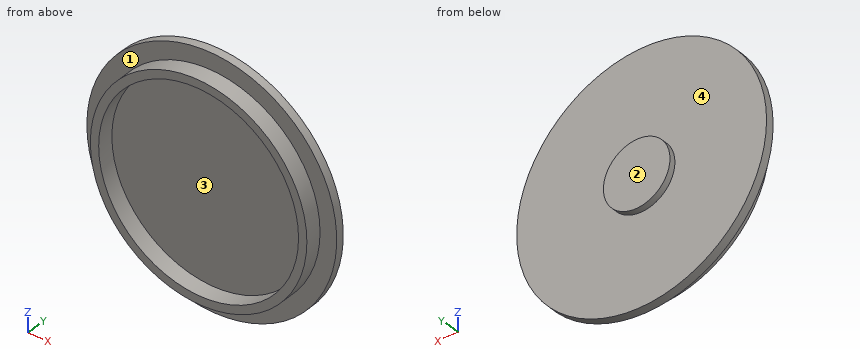
```python
from build123d import *


with BuildPart() as part:
    # Sketch1 → Lid Revolve (revolve)
    with BuildSketch(Plane.XY, mode=Mode.PRIVATE) as lid_revolve_sk:
        Polygon((0, 0), (48, 0), (48, -8), (52, -8), (52, 0), (60, 0), (60, 4), (16, 4), (16, 7), (0, 7), align=None)
    revolve(lid_revolve_sk.sketch.rotate(Axis((0, 7, 0), (0, -1, 0)), 180), axis=Axis((0, 7, 0), (0, -1, 0)))


solid = part.part
```
Input: part model. Units: mm. Frame: model coordinates. Face numbers are marked on the shaded views. A direction names the side the tool comes from. Give positions to 0.01 mm unless a question says otherwise; leave off trailing zeros. Order: outer loops, then holes, each group sorted by start corner. A loop starts at its lowest first (then second) coordinate and runs counter-clockwise, first axis right, second up. Notation, with made-up numbers: (32.5, -20) -> (87.5, -20) arc R29 ccw to (87.5, 2) -> close; hole circle Ø2 at (55.5, 64.5). An arc over 180 degrees is marked (long way). Write each question's results on one line, items separated by ' | '. Start each with the question number.
Item 1: Cut plane B-B on y = -3.5. Return the cut outline in (x, z).
Item 2: Cut plane C-C on z = 0. Return the cut outline in (x, y).
Item 3: Mould query, pull axis Z, two halves, no side actions, for the marked faces 3 and 4. Classes: pulls with the +Z half, pulls with the -Z half, needs draft (parallel to the pull), parting line crosses it, or undercut.
Item 4: Set-up query: the marked faces 1 and 2. Return all of +Z, -Z, +X, -X, +Y, -Y with unobstructed straight access to the full face (end or side cutting, diameter ignored); none if empty.
Item 5: Cut plane D-D on z = -35.5. Return the cut outline in (x, y).
Item 6: Line query: line 1 (Z direction, x = 0, y = -4.25); line 2 (Y direction, x = 34.5, z = 5.5); line 3 (Z direction, x = 18, y = -2). Output: solid intervals per line, ascending.
Item 7: Contact query for flat-ended pins moving along their axis: P1, Ø8, axis at y = 5, z = 27.5, coming from the -X side; P2, Ø5, axis at x = 1.5, z = -16, coming from the -Y side; P3, Ø6, axis at y = -5, z = 46, coming from the -X side. Output: stop coordinate, or through.
Item 8: Cut plane A-A on x = 0. Return the cut outline in (y, z).
Established:
1) outline: circle Ø104 at (0, 0); hole circle Ø96 at (0, 0)
2) outline: (-60, 0) -> (-52, 0) -> (-52, -8) -> (-48, -8) -> (-48, 0) -> (48, 0) -> (48, -8) -> (52, -8) -> (52, 0) -> (60, 0) -> (60, 4) -> (16, 4) -> (16, 7) -> (-16, 7) -> (-16, 4) -> (-60, 4) -> close
3) face 3: undercut | face 4: needs draft
4) face 1: -Y | face 2: +Z, -Z, +X, -X, +Y
5) outline: (-48.37, 0) -> (-38, 0) -> (-38, -8) -> (-32.31, -8) -> (-32.31, 0) -> (32.31, 0) -> (32.31, -8) -> (38, -8) -> (38, 0) -> (48.37, 0) -> (48.37, 4) -> (-48.37, 4) -> close
6) line 1: -52 to -48, 48 to 52 | line 2: 0 to 4 | line 3: -48.79 to -44.5, 44.5 to 48.79
7) P1: x = -55.15 | P2: y = 0 | P3: x = -29.24
8) outline: (-8, -52) -> (0, -52) -> (0, -60) -> (4, -60) -> (4, -16) -> (7, -16) -> (7, 16) -> (4, 16) -> (4, 60) -> (0, 60) -> (0, 52) -> (-8, 52) -> (-8, 48) -> (0, 48) -> (0, -48) -> (-8, -48) -> close
